Here's how the part is built. I have some questions about the finished solid (model axes, mm). A direction names the side the tool comes from. Give positions to 0.01 mm unless a question says otherwise; leave off trailing zeros. Write each loop counter-clockwise with the first axis right and the second up, starting at its lowest first coordinate (ties: lowest second). Pieces come first, ordered by that corner, then holes. Notation, with made-up numbers: (9.25, -30) -> (37.25, -30) arc R23 ccw to (37.25, -20) -> close; hole circle Ø10 at (57, 65.5). An arc over 180 degrees is marked (long way). Use one line per item in the form item = value.
```python
from build123d import *

# Parameters (mm, degrees)
MAIN_BODY_DEPTH                  = 3.81
CROSS_SCREW_BOSSES_DEPTH         = 31.75
F_8_CLEARANCE_HOLE1_D            = 4.4958
BALLOON_MONOFILAMENT_HOLE_D      = 2.5273
PARACHUTE_MONOFILAMENT_HOLE_D    = 2.5273
SKETCH21_W                       = 12.08
SKETCH21_H                       = 11.74
HOT_WIRE_CUTTER_HOLDER_DEPTH     = 9.67
CUT_EXTRUDE10_START              = -1.27
CUT_EXTRUDE10_DEPTH              = 63.383576094
CHAMFER8_SIZE                    = 0.381
SKETCH22_W                       = 6.029522694
SKETCH22_H                       = 1.524
SATELLITE_CABLE_MANAGEMENT_DEPTH = 66.050272386
SKETCH23_R                       = 3.175
BOSS_EXTRUDE7_DEPTH              = 20.066
SKETCH26_W                       = 6.35
SKETCH26_H                       = 6.35
CUT_EXTRUDE11_DEPTH              = 0.65024
CUT_EXTRUDE12_REACH              = 68.598
CUT_EXTRUDE12_END_RADIUS         = 3.3782
F_2_CLEARANCE_HOLE1_D            = 2.7051
F_2_CLEARANCE_HOLE1_DEPTH        = 3.175
TAP_DRILL_FOR_2_56_TAP1_D        = 1.778
TAP_DRILL_FOR_2_56_TAP1_DEPTH    = 3.175


with BuildPart() as part:
    # Sketch3 → Main body (new body)
    with BuildSketch(Plane.XY):
        with BuildLine():
            Line((-15.875, -38.1), (-15.875, 38.1))
            ThreePointArc((-15.875, 38.1), (-18.260491841, 42.291797068), (-23.082694008, 42.38179842))
            ThreePointArc((-23.082694008, 42.38179842), (-28.900226452, 38.649767283), (-34.12497326, 34.12497326))
            ThreePointArc((-34.12497326, 34.12497326), (-35.921024484, 34.12497326), (-35.921024484, 35.921024484))
            ThreePointArc((-35.921024484, 35.921024484), (0, 50.8), (35.921024484, 35.921024484))
            ThreePointArc((35.921024484, 35.921024484), (35.921024484, 34.12497326), (34.12497326, 34.12497326))
            ThreePointArc((34.12497326, 34.12497326), (28.900226452, 38.649767283), (23.082694008, 42.38179842))
            ThreePointArc((23.082694008, 42.38179842), (18.260491841, 42.291797068), (15.875, 38.1))
            Line((15.875, 38.1), (15.875, -38.1))
            ThreePointArc((15.875, -38.1), (18.260491841, -42.291797068), (23.082694008, -42.38179842))
            ThreePointArc((23.082694008, -42.38179842), (28.900226452, -38.649767283), (34.12497326, -34.12497326))
            ThreePointArc((34.12497326, -34.12497326), (35.921024484, -34.12497326), (35.921024484, -35.921024484))
            ThreePointArc((35.921024484, -35.921024484), (0, -50.8), (-35.921024484, -35.921024484))
            ThreePointArc((-35.921024484, -35.921024484), (-35.921024484, -34.12497326), (-34.12497326, -34.12497326))
            ThreePointArc((-34.12497326, -34.12497326), (-28.900226452, -38.649767283), (-23.082694008, -42.38179842))
            ThreePointArc((-23.082694008, -42.38179842), (-18.260491841, -42.291797068), (-15.875, -38.1))
        make_face()
    extrude(amount=MAIN_BODY_DEPTH)

    # Sketch5 → Cross screw bosses (add)
    with BuildSketch(Plane(origin=(15.875, 0, 0), x_dir=(0, 0, -1), z_dir=(1, 0, 0))):
        with BuildLine():
            Line((0, 38.1), (0, 26.99385))
            Line((0, 26.99385), (0, 14.29385))
            ThreePointArc((0, 14.29385), (1.86498297, 18.77886703), (6.35, 20.64385))
            ThreePointArc((6.35, 20.64385), (12.699998494, 26.998224058), (6.341251887, 33.343843974))
            ThreePointArc((6.341251887, 33.343843974), (2.338844583, 34.612930799), (0, 38.1))
        make_face()
        with BuildLine():
            ThreePointArc((6.261703048, -20.644463916), (1.864650947, -18.840779739), (0, -14.469233029))
            Line((0, -14.469233029), (0, -26.99385))
            Line((0, -26.99385), (0, -38.1))
            ThreePointArc((0, -38.1), (2.217611083, -34.670801888), (6.077775616, -33.338012189))
            ThreePointArc((6.077775616, -33.338012189), (6.213919542, -33.33945129), (6.35, -33.34385))
            ThreePointArc((6.35, -33.34385), (12.7, -26.99385), (6.35, -20.64385))
            ThreePointArc((6.35, -20.64385), (6.305852606, -20.644312569), (6.261703048, -20.644463916))
        make_face()
    extrude(amount=-CROSS_SCREW_BOSSES_DEPTH)

    # 8 Clearance Hole1 (through all)
    with Locations(Plane(origin=(15.875, 0, 0), x_dir=(0, 0, -1), z_dir=(1, 0, 0))):
        with Locations((6.35, 26.99385), (6.35, -26.893399733)):
            Hole(F_8_CLEARANCE_HOLE1_D / 2)

    # Balloon monofilament hole (through all)
    with Locations(Plane.XY.offset(3.81)):
        with Locations((-9.525, 0)):
            Hole(BALLOON_MONOFILAMENT_HOLE_D / 2)

    # Parachute monofilament hole (through all)
    with Locations(Plane.XY.offset(3.81)):
        with Locations((9.525, 0)):
            Hole(PARACHUTE_MONOFILAMENT_HOLE_D / 2)

    # Sketch21 → Hot wire cutter holder (add)
    with BuildSketch(Plane.XY.offset(-8.5979)):
        with Locations((-5.315, -27.056)):
            Rectangle(SKETCH21_W, SKETCH21_H)
    extrude(amount=-HOT_WIRE_CUTTER_HOLDER_DEPTH)

    # Sketch21_10 → Cut-Extrude10 (cut, through all)
    with BuildSketch(Plane.XY.offset(-8.5979).offset(CUT_EXTRUDE10_START)):
        with BuildLine():
            Line((-4.243, -30.386), (-2.315, -30.386))
            ThreePointArc((-2.315, -30.386), (-1.961446609, -30.239553391), (-1.815, -29.886))
            Line((-1.815, -29.886), (-1.815, -24.786))
            Line((-1.815, -24.786), (-1.765, -24.786))
            ThreePointArc((-1.765, -24.786), (-1.623578644, -24.727421356), (-1.565, -24.586))
            Line((-1.565, -24.586), (-1.565, -24.386))
            Line((-1.565, -24.386), (-1.815, -24.386))
            Line((-1.815, -24.386), (-1.815, -21.186))
            Line((-1.815, -21.186), (-8.815, -21.186))
            Line((-8.815, -21.186), (-8.815, -30.386))
            Line((-8.815, -30.386), (-7.418, -30.386))
            Line((-7.418, -30.386), (-7.418, -32.926))
            Line((-7.418, -32.926), (-4.243, -32.926))
            Line((-4.243, -32.926), (-4.243, -30.386))
        make_face()
    extrude(amount=-CUT_EXTRUDE10_DEPTH, mode=Mode.SUBTRACT)

    # Chamfer8
    chamfer8_edges = [part.edges().sort_by_distance(p)[0] for p in [
        (-8.1165, -30.386, -18.2679),
        (-8.815, -25.786, -18.2679),
        (-3.279, -30.386, -18.2679),
        (-1.961446609, -30.239553391, -18.2679),
        (-1.815, -27.336, -18.2679),
    ]]
    chamfer(chamfer8_edges, length=CHAMFER8_SIZE)

    # Sketch22 → satellite cable management (cut, through all)
    with BuildSketch(Plane(origin=(0, 0, 0), x_dir=(-1, 0, 0), z_dir=(0, 0, -1))):
        with Locations((0, -47.038383029)):
            Rectangle(SKETCH22_W, SKETCH22_H)
        with Locations((0, -41.958383029)):
            Rectangle(SKETCH22_W, SKETCH22_H)
    extrude(amount=-SATELLITE_CABLE_MANAGEMENT_DEPTH, mode=Mode.SUBTRACT)

    # Sketch23 → Boss-Extrude7 (add)
    with BuildSketch(Plane(origin=(0, 0, 0), x_dir=(-1, 0, 0), z_dir=(0, 0, -1))):
        Polygon((-8.490181608, 45.085), (1.161818392, 45.085), (1.161818392, 38.735), (-8.490181608, 38.735), (-8.490181608, 35.56), (11.829818392, 35.56), (11.829818392, 48.26), (-8.490181608, 48.26), align=None)
        with Locations((5.479818392, 41.91)):
            Circle(SKETCH23_R, mode=Mode.SUBTRACT)
    extrude(amount=BOSS_EXTRUDE7_DEPTH)

    # Sketch25 → 1_4 QR pin hole (revolve, cut)
    with BuildSketch(Plane(origin=(-5.479818392, 41.91, -20.066), x_dir=(0, 1, 0), z_dir=(1, 0, 0))):
        Polygon((0, 0), (0, 23.876), (4.0132, 23.876), (3.3782, 23.241), (3.3782, 0), align=None)
    revolve(axis=Axis((-5.479818392, 41.91, -26.416), (0, 0, 1)), mode=Mode.SUBTRACT)

    # Sketch26 → Cut-Extrude11 (cut)
    with BuildSketch(Plane(origin=(-1.161818392, 0, 0), x_dir=(0, 0, -1), z_dir=(1, 0, 0))):
        with Locations((7.366, 41.91)):
            Rectangle(SKETCH26_W, SKETCH26_H)
    extrude(amount=-CUT_EXTRUDE11_DEPTH, mode=Mode.SUBTRACT)

    # Cut-Extrude12: up to this cylinder (the profile starts outside it)
    cut_extrude12_end = Plane(origin=(-5.479818392, 41.91, -7.366), z_dir=(0, 0, -1)) * Cylinder(CUT_EXTRUDE12_END_RADIUS, 146.095802, mode=Mode.PRIVATE)
    # Sketch27 → Cut-Extrude12 (cut, up to the surface)
    with BuildSketch(Plane(origin=(-1.812058392, 0, 0), x_dir=(0, 0, -1), z_dir=(1, 0, 0)), mode=Mode.PRIVATE) as cut_extrude12_sk1:
        with BuildLine():
            ThreePointArc((9.271, 41.91), (9.125990509, 42.639011939), (8.713038418, 43.257038418))
            Line((8.713038418, 43.257038418), (6.018961582, 40.562961582))
            ThreePointArc((6.018961582, 40.562961582), (8.095011939, 40.150009491), (9.271, 41.91))
        make_face()
    cut_extrude12_tool1 = extrude(cut_extrude12_sk1.sketch, amount=-CUT_EXTRUDE12_REACH, mode=Mode.PRIVATE) - cut_extrude12_end
    add(cut_extrude12_tool1.solids().sort_by_distance((-1.812058, 41.338299, -7.937701))[0], mode=Mode.SUBTRACT)
    # Sketch27 → Cut-Extrude12 (cut, up to the surface)
    with BuildSketch(Plane(origin=(-1.812058392, 0, 0), x_dir=(0, 0, -1), z_dir=(1, 0, 0)), mode=Mode.PRIVATE) as cut_extrude12_sk2:
        with BuildLine():
            Line((6.018961582, 40.562961582), (8.713038418, 43.257038418))
            ThreePointArc((8.713038418, 43.257038418), (6.018961582, 43.257038418), (6.018961582, 40.562961582))
        make_face()
    cut_extrude12_tool2 = extrude(cut_extrude12_sk2.sketch, amount=-CUT_EXTRUDE12_REACH, mode=Mode.PRIVATE) - cut_extrude12_end
    add(cut_extrude12_tool2.solids().sort_by_distance((-1.812058, 42.481701, -6.794299))[0], mode=Mode.SUBTRACT)
    # Sketch27 → Cut-Extrude12 (cut, up to the surface)
    with BuildSketch(Plane(origin=(-1.812058392, 0, 0), x_dir=(0, 0, -1), z_dir=(1, 0, 0)), mode=Mode.PRIVATE) as cut_extrude12_sk3:
        with BuildLine():
            ThreePointArc((9.271, 41.91), (9.125990509, 42.639011939), (8.713038418, 43.257038418))
            Line((8.713038418, 43.257038418), (6.018961582, 40.562961582))
            ThreePointArc((6.018961582, 40.562961582), (8.095011939, 40.150009491), (9.271, 41.91))
        make_face()
    cut_extrude12_tool3 = extrude(cut_extrude12_sk3.sketch, amount=-CUT_EXTRUDE12_REACH, mode=Mode.PRIVATE) - cut_extrude12_end
    add(cut_extrude12_tool3.solids().sort_by_distance((-1.812058, 41.338299, -7.937701))[0], mode=Mode.SUBTRACT)
    # Sketch27 → Cut-Extrude12 (cut, up to the surface)
    with BuildSketch(Plane(origin=(-1.812058392, 0, 0), x_dir=(0, 0, -1), z_dir=(1, 0, 0)), mode=Mode.PRIVATE) as cut_extrude12_sk4:
        with BuildLine():
            Line((6.018961582, 40.562961582), (8.713038418, 43.257038418))
            ThreePointArc((8.713038418, 43.257038418), (6.018961582, 43.257038418), (6.018961582, 40.562961582))
        make_face()
    cut_extrude12_tool4 = extrude(cut_extrude12_sk4.sketch, amount=-CUT_EXTRUDE12_REACH, mode=Mode.PRIVATE) - cut_extrude12_end
    add(cut_extrude12_tool4.solids().sort_by_distance((-1.812058, 42.481701, -6.794299))[0], mode=Mode.SUBTRACT)

    # 2 Clearance Hole1
    with Locations(Plane(origin=(0, 48.26, 0), x_dir=(1, 0, 0), z_dir=(0, 1, 0))):
        with Locations((5.315181608, 5.08), (5.315181608, 14.605)):
            Hole(F_2_CLEARANCE_HOLE1_D / 2, depth=F_2_CLEARANCE_HOLE1_DEPTH)

    # Tap Drill for _2-56 Tap1
    with Locations(Plane(origin=(0, 38.735, 0), x_dir=(1, 0, 0), z_dir=(0, 1, 0))):
        with Locations((5.315181608, 14.605), (5.315181608, 5.08)):
            Hole(TAP_DRILL_FOR_2_56_TAP1_D / 2, depth=TAP_DRILL_FOR_2_56_TAP1_DEPTH)


solid = part.part
```
Q1. Will these pins go through, and if not, where does the flat tip stop? pin 1 Ø0.5 at (y, z) = (-42, 2.5) entering from +X; pin 2 Ø1.2 at (y, z) = (-47.5, 1.5) entering from -X; pin 3 Ø8 at (x, z) = (-2.5, -3.5) entering from -Y.
Result set:
pin_1 = 28.94
pin_2 = -19.52
pin_3 = -50.8
Q2. If I drill on line 1 along Y through (x, z) = (-6, -6); line 2 along X through (y, z) = (36, 0.25) (3 decimals); line 3 along Y through (x, z) = (-7, -5), over which ranges is the centre line in solid material (lowest first)? Write a range as from..to.
Result set:
line_1 = -33.34..-29.11, -24.67..-20.64, 20.63..24.77, 29.21..33.34, 35.56..38.57, 45.25..48.26
line_2 = -35.842..-32.141, -15.875..15.875, 32.141..35.842
line_3 = -33.43..-28.69, -25.1..-20.52, 20.5..25.2, 28.79..33.45, 35.56..38.89, 44.93..48.26
Q3. I want a section at C-C, the plane y = 16.5. Write out the boundary of the cut face in (x, z) (3 decimals), and give its area (3 significant figures).
Result set:
outline = (-15.875, -0.401) -> (15.875, -0.401) -> (15.875, 3.81) -> (-15.875, 3.81) -> close
area = 134 mm2
Q4. I want a section at B-B, the plane x = 17.5. Write out the boundary of the cut face in (y, z), and give its area (3 significant figures).
Result set:
outline = (-47.69, 0) -> (-41.73, 0) -> (-41.73, 3.81) -> (-47.69, 3.81) -> close; (41.73, 0) -> (47.69, 0) -> (47.69, 3.81) -> (41.73, 3.81) -> close
area = 45.4 mm2
Q5. I want a section at D-D, the plane y = -17.5. Write out the boundary of the cut face in (x, z) (3 decimals).
Result set:
outline = (-15.875, -0.831) -> (15.875, -0.831) -> (15.875, 3.81) -> (-15.875, 3.81) -> close
Q6. I want a section at A-A, the plane y = 0. Write out the boundary of the cut face in (x, z) (3 decimals), and give its area (3 significant figures).
Result set:
outline = (-15.875, 0) -> (-10.789, 0) -> (-10.789, 3.81) -> (-15.875, 3.81) -> close; (-8.261, 0) -> (8.261, 0) -> (8.261, 3.81) -> (-8.261, 3.81) -> close; (10.789, 0) -> (15.875, 0) -> (15.875, 3.81) -> (10.789, 3.81) -> close
area = 102 mm2
Q7. Which directions (+Z, -Z, +X, -X, +Y, -Y) give clear straight access to the entire face, cutting with the end or side of a thin tool? Please do faces 4 (the face through (-5.4, -21.186, -9.4)), 5 (the face through (-3, -30.386, -14)), 6 (the face through (28.82, -38.71, 1.88)).
Result set:
face_4 = -Z, +X, -X
face_5 = -Z
face_6 = +Z, -Z
Q8. If we mould it in two halves opening along Y, with no side actions, what happens to faces 1 (the face through (-0.559, 50.797, 1.878)), 2 (the face through (0, 0, 0)), 3 (the face through (6.4, 46.7, -13.8))? For each: +Y half, -Y half, draft (parallel to the pull), parting line (faces both ways), or undercut.
Result set:
face_1 = +Y half
face_2 = undercut
face_3 = draft
